from build123d import *

# Parameters (mm, degrees)
EXTRUDE_THIN1_DEPTH = 381
FILLET1_R           = 0.889


with BuildPart() as part:
    # Sketch1 → Extrude-Thin1 (new body)
    with BuildSketch(Plane.XY):
        Polygon((-1.285875, 3.175), (0, 0), (-3.175, 0), (-9.525, 7.9375), (-9.525, 14.2875), (-1.285875, 14.2875), (-1.285875, 23.8125), (-9.525, 23.8125), (-9.525, 30.1625), (-3.175, 38.1), (0, 38.1), (-1.285875, 34.925), (-2.109862469, 35.258714925), (-1.319187013, 37.211), (-2.747724511, 37.211), (-8.636, 29.850655638), (-8.636, 24.7015), (-0.396875, 24.7015), (-0.396875, 13.3985), (-8.636, 13.3985), (-8.636, 8.249344362), (-2.747724511, 0.889), (-1.319187013, 0.889), (-2.109862469, 2.841285075), align=None)
    extrude(amount=-EXTRUDE_THIN1_DEPTH)

    # Fillet1
    fillet1_edges = [part.edges().sort_by_distance(p)[0] for p in [
        (-3.175, 0, -190.5),
        (-9.525, 7.9375, -190.5),
        (-9.525, 14.2875, -190.5),
        (-9.525, 23.8125, -190.5),
        (-9.525, 30.1625, -190.5),
        (-3.175, 38.1, -190.5),
        (-0.396875, 24.7015, -190.5),
        (-0.396875, 13.3985, -190.5),
    ]]
    fillet(fillet1_edges, radius=FILLET1_R)


solid = part.part
Here's how the part is built. I have some questions about the finished solid (model axes, mm). A direction names the side the tool comes from. Round coordinates to 2 decimals unless told otherwise and drop trailing zeros. Loops run counter-clockwise (first coordinate to the right, second up) from the corner with the lowest first, then second, coordinate; pieces in that order, holes last.
1. If I drill on line 1 along Y through (x, z) = (-2.25, -255); line 2 along Y through (x, z) = (-5.5, -151); line 3 along Y through (x, z) = (-1.5, -196.5), over which ranges is the centre line in solid material (lowest first)?
Answer list:
line 1: y = 0 to 0.89, 13.4 to 14.29, 23.81 to 24.7, 37.21 to 38.1
line 2: y = 2.91 to 4.33, 13.4 to 14.29, 23.81 to 24.7, 33.77 to 35.19
line 3: y = 0 to 0.89, 1.34 to 3.09, 13.4 to 14.29, 23.81 to 24.7, 35.01 to 36.76, 37.21 to 38.1
2. If we section it at B-B on x = -7: Write out the boundary of the cut face in (y, z), plus the area to 3 significant figures.
Answer list:
outline: (4.78, -381) - (6.2, -381) - (6.2, 0) - (4.78, 0) - close; (13.4, -381) - (14.29, -381) - (14.29, 0) - (13.4, 0) - close; (23.81, -381) - (24.7, -381) - (24.7, 0) - (23.81, 0) - close; (31.9, -381) - (33.32, -381) - (33.32, 0) - (31.9, 0) - close
area: 1,760 mm2
3. Which directions (+Z, -Z, +X, -X, +Y, -Y) give clear straight access to the entire face, cutting with the end or side of a thin tool? Please do faces 1 (the face through (-1, 18, 0)), 2 (the face through (-5, 14.288, -188)), 3 (the face through (-5.65, 33.58, -187.83)), 4 (the face through (-1, 18, -381)), 5 (the face through (-5, 13.398, -188)).
Answer list:
face 1: +Z, +X, -X, +Y, -Y
face 2: +Z, -Z, -X
face 3: +Z, -Z
face 4: -Z, +X, -X, +Y, -Y
face 5: +Z, -Z, +X
4. We'd pull the mould along Y, two halves only. Please class faces 6 (the face through (-5.73, 4.62, -187.83)), 7 (the face through (-6.43, 34.03, -187.83)), 8 (the face through (-1.286, 19, -188)), 9 (the face through (-6.345, 3.962, -187.833)): +Y half, -Y half, draft (parallel to the pull), parting line (faces both ways), or undercut.
Answer list:
face 6: undercut
face 7: +Y half
face 8: undercut
face 9: -Y half
5. For P1, Ø3.5, axis at x = -3.5, z = -249, coming from the +Y side; P2, Ø3, axis at y = 17.5, z = -95.5, coming from the +X side; P3, Ø5.5, axis at y = 28.5, z = -272.5, coming from the +X side; P4, Ø3.5, axis at x = -6.5, z = -269.5, coming from the +Y side, each with a flat end and sliding along its axis, tell me the tip position at first contact or that it passes through.
Answer list:
P1: stops at y = 38.1
P2: stops at x = -0.4
P3: stops at x = -7.52
P4: stops at y = 36.13
